```python
from build123d import *

# Parameters (mm, degrees)
SKETCH2_R              = 2.074585303
VSLOT2020_2020_5_DEPTH = 254


with BuildPart() as part:
    # Sketch2 → Vslot2020 2020(5) (new body)
    with BuildSketch(Plane.ZX):
        with BuildLine():
            Line((13.9, 7.149086807), (13.9, 12.844511469))
            Line((13.9, 12.844511469), (16.558493656, 15.492177728))
            Line((16.558493656, 15.492177728), (16.550703242, 15.5))
            Line((16.550703242, 15.5), (18.2, 15.5))
            Line((18.2, 15.5), (18.2, 13.12))
            Line((18.2, 13.12), (18.534428266, 13.12))
            Line((18.534428266, 13.12), (20, 14.58))
            Line((20, 14.58), (20, 19.5))
            ThreePointArc((20, 19.5), (19.853553391, 19.853553391), (19.5, 20))
            Line((19.5, 20), (14.575, 20))
            Line((14.575, 20), (13.12, 18.545))
            Line((13.12, 18.545), (13.12, 18.2))
            Line((13.12, 18.2), (15.5, 18.2))
            Line((15.5, 18.2), (15.5, 16.555))
            Line((15.5, 16.555), (12.834142613, 13.9))
            Line((12.834142613, 13.9), (7.155, 13.9))
            Line((7.155, 13.9), (4.5, 16.555))
            Line((4.5, 16.555), (4.5, 18.2))
            Line((4.5, 18.2), (6.875, 18.2))
            Line((6.875, 18.2), (6.875, 18.545))
            Line((6.875, 18.545), (5.42, 20))
            Line((5.42, 20), (0.5, 20))
            ThreePointArc((0.5, 20), (0.146446609, 19.853553391), (0, 19.5))
            Line((0, 19.5), (0, 14.58))
            Line((0, 14.58), (1.46, 13.12))
            Line((1.46, 13.12), (1.8, 13.12))
            Line((1.8, 13.12), (1.8, 15.5))
            Line((1.8, 15.5), (3.445, 15.5))
            Line((3.445, 15.5), (3.439339828, 15.494339828))
            Line((3.439339828, 15.494339828), (6.094339828, 12.839339828))
            Line((6.094339828, 12.839339828), (6.1, 12.845))
            Line((6.1, 12.845), (6.1, 7.149086807))
            Line((6.1, 7.149086807), (3.439339828, 4.5))
            Line((3.439339828, 4.5), (1.8, 4.5))
            Line((1.8, 4.5), (1.8, 6.88))
            Line((1.8, 6.88), (1.46, 6.88))
            Line((1.46, 6.88), (0, 5.42))
            Line((0, 5.42), (0, 0.5))
            ThreePointArc((0, 0.5), (0.146446609, 0.146446609), (0.5, 0))
            Line((0.5, 0), (5.42, 0))
            Line((5.42, 0), (6.875, 1.455))
            Line((6.875, 1.455), (6.875, 1.8))
            Line((6.875, 1.8), (4.5, 1.8))
            Line((4.5, 1.8), (4.5, 3.4393348))
            Line((4.5, 3.4393348), (7.158345795, 6.086117297))
            Line((7.158345795, 6.086117297), (7.144523479, 6.1))
            Line((7.144523479, 6.1), (12.854625295, 6.1))
            Line((12.854625295, 6.1), (12.841221344, 6.086548451))
            Line((12.841221344, 6.086548451), (15.499715, 3.437461644))
            Line((15.499715, 3.437461644), (15.5, 1.8))
            Line((15.5, 1.8), (13.12, 1.8))
            Line((13.12, 1.8), (13.12, 1.455))
            Line((13.12, 1.455), (14.575, 0))
            Line((14.575, 0), (19.5, 0))
            ThreePointArc((19.5, 0), (19.853553391, 0.146446609), (20, 0.5))
            Line((20, 0.5), (20, 5.42))
            Line((20, 5.42), (18.606904708, 6.88))
            Line((18.606904708, 6.88), (18.2, 6.88))
            Line((18.2, 6.88), (18.2, 4.5))
            Line((18.2, 4.5), (16.558493656, 4.5))
            Line((16.558493656, 4.5), (13.9, 7.149086807))
        make_face()
        with Locations((10, 10)):
            Circle(SKETCH2_R, mode=Mode.SUBTRACT)
    extrude(amount=VSLOT2020_2020_5_DEPTH)


solid = part.part
```
Source: CAD feature listing. Evaluate the final solid. Frame: model axes, mm. A direction names the side the tool comes from. Coordinates: 2 decimals unless noted, no trailing zeros. Loops run counter-clockwise (first coordinate to the right, second up) from the corner with the lowest first, then second, coordinate; pieces in that order, holes last. Notation, with made-up numbers: M -18.5,31.25 L -6.5,31.25 A8 ccw -6.5,45.25 Z; hole C 6.25,82.25 d1. An arc over 180 degrees is marked long. Use a Markdown table: item, result. Add a question column.
Q1. First-contact query: pin 1 (1 mm diameter, centred on x = 6.5, y = 135, fed in from +Z); pin 2 (3 mm diameter, centred on x = 9.5, y = 76.5, fed in from +Z); pin 3 (6 mm diameter, centred on y = 174, z = 10.5, fed in from -X) (3 decimals). Flat tips, straight axial feed; report the tip coordinate or a pass-through.
Q2. Draft query along Z for faces 1 (the flat face through (10, 125, 13.9)), 2 (the flat face through (10.1, 254, 7.6)), 3 (the flat face through (13.9, 125, 10)). Return one class per face: pulls with the +Z half, pulls with the -Z half, needs draft (parallel to the pull), parting line crosses it, or undercut.
Q3. Section query B-B, the plane z = 10. Return loops of the section in (x, y), and give its area (3 significant figures).
Q4. Access query for faces 4 (the flat face through (0, 125, 17)), 5 (the flat face through (10, 125, 6.1)), 6 (the flat face through (6.1, 125, 10)). Directions: +Z, -Z, +X, -X, +Y, -Y. A direction counts if a zero-diameter tool reaches every point of the face in a straight line with its end or side. Return the directions, or none.
Q5. Section query A-A, the plane x = 10. Return loops of the section in (y, z).
Q6. Material intervals for L1, parallel to Z at x = 2.5, y = 73; L2, parallel to X at y = 98.5, z = 10, sorted ascending.
Result:
| question | item | result |
|---|---|---|
| 1 | pin 1 | stops at z = 19.45 |
| 1 | pin 2 | stops at z = 13.9 |
| 1 | pin 3 | stops at x = 1.075 |
| 2 | face 1 | pulls with the +Z half |
| 2 | face 2 | needs draft |
| 2 | face 3 | undercut |
| 3 | outline | M 6.1,0 L 7.93,0 L 7.93,254 L 6.1,254 Z; M 12.07,0 L 13.9,0 L 13.9,254 L 12.07,254 Z |
| 3 | area | 927 mm2 |
| 4 | face 4 | +Z, -Z, -X, +Y, -Y |
| 4 | face 5 | -Z, +Y, -Y |
| 4 | face 6 | -X, +Y, -Y |
| 5 | outline | M 0,6.1 L 254,6.1 L 254,7.93 L 0,7.93 Z; M 0,12.07 L 254,12.07 L 254,13.9 L 0,13.9 Z |
| 6 | L1 | z = 0 to 4.5, 15.5 to 20 |
| 6 | L2 | x = 6.1 to 7.93, 12.07 to 13.9 |
